Verification items for the finished model (mm, model axes). A direction names the side the tool comes from. Round coordinates to 2 decimals unless told otherwise and drop trailing zeros. Loops run counter-clockwise (first coordinate to the right, second up) from the corner with the lowest first, then second, coordinate; pieces in that order, holes last. Notation, with made-up numbers: (31, 17.5) - (37, 17.5) arc R24 ccw to (37, 47.5) - close; hole circle Ø4 at (-13, 40). An arc over 180 degrees is marked (long way). Use a Markdown table: item, result. Add a question column.
```python
from build123d import *

# Parameters (mm, degrees)
SKETCH1_W                    = 8
SKETCH1_H                    = 16.7
BASE_FLANGE1_DEPTH           = 0.2
EDGE_FLANGE2_STRIP_W         = 2.2732
EDGE_FLANGE2_STRIP_H         = 0.2
EDGE_FLANGE2_STRIP_CUT_DEPTH = 8
EDGE_FLANGE2_DEPTH           = 8
EDGE_FLANGE3_STRIP_CUT_DEPTH = 8
EDGE_FLANGE3_DEPTH           = 8
HEM1_START                   = -4
HEM1_DEPTH                   = 8
EDGE_FLANGE4_START           = -4
EDGE_FLANGE4_DEPTH           = 8
EDGE_FLANGE5_STRIP_W         = 2.2732
EDGE_FLANGE5_STRIP_H         = 0.2
EDGE_FLANGE5_STRIP_CUT_DEPTH = 8
EDGE_FLANGE5_DEPTH           = 8
FILLET1_R                    = 1


# Read off the part's stored shape, not the designer's step: Hem1, Edge-Flange4
# Sheet-metal steps are written as plain solids
with BuildPart() as part:
    # Sketch1 → Base-Flange1 (new body)
    with BuildSketch(Plane(origin=(0, 0, 0), x_dir=(1, 0, 0), z_dir=(0, 1, 0))):
        with Locations((0, 8.35)):
            Rectangle(SKETCH1_W, SKETCH1_H)
    extrude(amount=BASE_FLANGE1_DEPTH)

    # Edge-Flange2 strip (across the edge) → Edge-Flange2 strip cut (cut)
    with BuildSketch(Plane(origin=(4, 0, 0), x_dir=(0, 0, -1), z_dir=(-1, 0, 0))):
        with Locations((-0.4, -0.1)):
            Rectangle(EDGE_FLANGE2_STRIP_W, EDGE_FLANGE2_STRIP_H)
    extrude(amount=EDGE_FLANGE2_STRIP_CUT_DEPTH, mode=Mode.SUBTRACT)

    # Edge-Flange2 section (across the edge) → Edge-Flange2 (add)
    with BuildSketch(Plane(origin=(4, 0, 0), x_dir=(0, 0, -1), z_dir=(-1, 0, 0))):
        with BuildLine():
            Line((-0.2, 0.7366), (-0.2, 8.3))
            Line((-0.2, 8.3), (0, 8.3))
            Line((0, 8.3), (0, 0.7366))
            ThreePointArc((0, 0.7366), (0.215745145, 0.215745145), (0.7366, 0))
            Line((0.7366, 0), (0.7366, -0.2))
            ThreePointArc((0.7366, -0.2), (0.074323789, 0.074323789), (-0.2, 0.7366))
        make_face()
    extrude(amount=EDGE_FLANGE2_DEPTH)

    # Edge-Flange3 strip (across the edge) → Edge-Flange3 strip cut (cut)
    with BuildSketch(Plane(origin=(4, -8.3, 0), x_dir=(0, 0.8660254037844346, -0.5000000000000071), z_dir=(-1, 0, 0))):
        Polygon((-1.700348948, 0.750756815), (0.2683, -0.385843185), (0.3683, -0.212638104), (-1.600348948, 0.923961896), align=None)
    extrude(amount=EDGE_FLANGE3_STRIP_CUT_DEPTH, mode=Mode.SUBTRACT)

    # Edge-Flange3 section (across the edge) → Edge-Flange3 (add)
    with BuildSketch(Plane(origin=(4, -8.3, 0), x_dir=(0, 0.8660254037844346, -0.5000000000000071), z_dir=(-1, 0, 0))):
        with BuildLine():
            Line((-0.2, 0.425276208), (-0.2, 0.984529946))
            Line((-0.2, 0.984529946), (0, 0.984529946))
            Line((0, 0.984529946), (0, 0.425276208))
            ThreePointArc((0, 0.425276208), (0.098685688, 0.056976208), (0.3683, -0.212638104))
            Line((0.3683, -0.212638104), (0.2683, -0.385843185))
            ThreePointArc((0.2683, -0.385843185), (-0.074519393, -0.043023792), (-0.2, 0.425276208))
        make_face()
    extrude(amount=EDGE_FLANGE3_DEPTH)

    # Hem1 outline → Hem1 (add)
    with BuildSketch(Plane.YZ.offset(HEM1_START)):
        with BuildLine():
            Line((-8.701650804, 1.012627873), (-8.506776791, 1.057618084))
            ThreePointArc((-8.506776791, 1.057618084), (-13.680298712, 0.854349855), (-8.792264973, -0.852627944))
            Line((-8.792264973, -0.852627944), (-8.965470054, -0.752627944))
            ThreePointArc((-8.965470054, -0.752627944), (-13.482495539, 0.824787973), (-8.701650804, 1.012627873))
        make_face()
    extrude(amount=HEM1_DEPTH)

    # Edge-Flange4 outline → Edge-Flange4 (add)
    with BuildSketch(Plane.YZ.offset(EDGE_FLANGE4_START)):
        with BuildLine():
            ThreePointArc((-8.701650804, 1.012627873), (-8.37210301, 0.490326231), (-7.789055802, 0.286717031))
            Line((-7.789055802, 0.286717031), (0.285026102, 0.286717031))
            Line((0.285026102, 0.286717031), (0.285026102, 0.486717031))
            Line((0.285026102, 0.486717031), (-7.789055802, 0.486717031))
            ThreePointArc((-7.789055802, 0.486717031), (-8.247600083, 0.646847862), (-8.506776791, 1.057618084))
            Line((-8.506776791, 1.057618084), (-8.701650804, 1.012627873))
        make_face()
    extrude(amount=EDGE_FLANGE4_DEPTH)

    # Edge-Flange5 strip (across the edge) → Edge-Flange5 strip cut (cut)
    with BuildSketch(Plane(origin=(-4, 0.285026102, 0.286717031), x_dir=(0, -1, 0), z_dir=(1, 0, 0))):
        with Locations((-0.4, -0.1)):
            Rectangle(EDGE_FLANGE5_STRIP_W, EDGE_FLANGE5_STRIP_H)
    extrude(amount=EDGE_FLANGE5_STRIP_CUT_DEPTH, mode=Mode.SUBTRACT)

    # Edge-Flange5 section (across the edge) → Edge-Flange5 (add)
    with BuildSketch(Plane(origin=(-4, 0.285026102, 0.286717031), x_dir=(0, -1, 0), z_dir=(1, 0, 0))):
        with BuildLine():
            Line((-0.2, 0.7366), (-0.2, 16.4))
            Line((-0.2, 16.4), (0, 16.4))
            Line((0, 16.4), (0, 0.7366))
            ThreePointArc((0, 0.7366), (0.215745145, 0.215745145), (0.7366, 0))
            Line((0.7366, 0), (0.7366, -0.2))
            ThreePointArc((0.7366, -0.2), (0.074323789, 0.074323789), (-0.2, 0.7366))
        make_face()
    extrude(amount=EDGE_FLANGE5_DEPTH)

    # Fillet1
    fillet1_edges = [part.edges().sort_by_distance(p)[0] for p in [
        (-4, 0.385026102, -16.113282969),
        (4, 0.385026102, -16.113282969),
        (-4, 0.1, -16.7),
        (4, 0.1, -16.7),
    ]]
    fillet(fillet1_edges, radius=FILLET1_R)


solid = part.part
```
Q1. Set-up check for faces 5 (the face through (-0.056, -8.379, 0.496)), 6 (the face through (0, -4, 0.487)), 7 (the face through (0, 0.485, -8)): record each of +Z, -Z, +X, -X, +Y, -Y from which the full face is reachable in a straight line by a thin tool's end or side.
Q2. Section check D-D on z = -1.5. Record the cut outline in (x, y).
Q3. Section check C-C on x = -1.5. Record the cut outline in (y, z) (3 decimals).
Q4. Thickness scan on line 1 along Z through (x, y) = (-2.25, -11); line 2 along Z through (x, y) = (-2.5, -10); line 3 along Y through (x, z) = (-2, 2). Record the ranges inside material, lowest first.
Q5. Release check for a two-part mould opening along Z. For faces 1 (the face through (-0.056, -13.663, 0.955)), 2 (the face through (-0.056, -13.495, 0.731)), 3 (the face through (0, 0, -9)), 4 (the face through (0, -4, 0)) record: +Z half, -Z half, draft (parallel to the pull), parting line (faces both ways), or undercut.
Q6. Section check A-A on y = -4. Record the cut outline in (x, z), plus the area to 3 significant figures.
Q7. Go/stop test with flat-tipped pins: pin 1 Ø3 at (x, y) = (-1.5, -1.5) entering from +Z; pin 2 Ø2 at (x, y) = (0, -4) entering from -Z; pin 3 Ø2 at (x, z) = (-3, -7.5) entering from -Y; pin 4 Ø5 at (y, z) = (-2, -11) entering from +X. Record where each tip stops, or that it passes through.
Determined:
| question | item | result |
|---|---|---|
| 1 | face 5 | +X, -X |
| 1 | face 6 | +Z, +X, -X, +Y |
| 1 | face 7 | +Z, -Z, +X, -X, +Y |
| 2 | outline | (-4, -12.83) - (4, -12.83) - (4, -12.51) - (-4, -12.51) - close; (-4, -9.64) - (4, -9.64) - (4, -9.32) - (-4, -9.32) - close; (-4, 0) - (4, 0) - (4, 0.2) - (-4, 0.2) - close; (-4, 0.29) - (4, 0.29) - (4, 0.49) - (-4, 0.49) - close |
| 3 | outline | (-8.965, -0.753) arc R2.435 cw (long way) to (-8.702, 1.013) arc R0.937 ccw to (-7.789, 0.287) - (-0.452, 0.287) arc R0.737 cw to (0.285, -0.45) - (0.285, -16.113) - (0.485, -16.113) - (0.485, -0.45) arc R0.937 ccw to (-0.452, 0.487) - (-7.789, 0.487) arc R0.737 cw to (-8.507, 1.058) arc R2.635 ccw (long way) to (-8.792, -0.853) - (-8.513, -0.368) arc R0.737 cw to (-7.875, 0) - (-0.737, 0) arc R0.737 cw to (0, -0.737) - (0, -16.7) - (0.2, -16.7) - (0.2, -0.737) arc R0.937 ccw to (-0.737, 0.2) - (-7.875, 0.2) arc R0.937 ccw to (-8.686, -0.268) - close |
| 4 | line 1 | z = -2.17 to -1.97, 2.9 to 3.1 |
| 4 | line 2 | z = -1.94 to -1.72, 2.65 to 2.87 |
| 4 | line 3 | y = -13.22 to -12.96, -9.18 to -8.93 |
| 5 | face 1 | parting line |
| 5 | face 2 | undercut |
| 5 | face 3 | draft |
| 5 | face 4 | -Z half |
| 6 | outline | (-4, 0) - (4, 0) - (4, 0.2) - (-4, 0.2) - close; (-4, 0.29) - (4, 0.29) - (4, 0.49) - (-4, 0.49) - close |
| 6 | area | 3.20 mm² |
| 7 | pin 1 | stops at z = 0.49 |
| 7 | pin 2 | stops at z = 0 |
| 7 | pin 3 | stops at y = 0 |
| 7 | pin 4 | stops at x = 4 |
